Geometry check sheet. Reference: drawing and pictorial views, mm from the part's lowest x, y, z. A direction names the side the tool comes from. Round coordinates to 2 decimals unless told otherwise and drop trailing zeros. Order: outer loops, then holes, each group sorted by start corner. A loop starts at its lowest first (then second) coordinate and runs counter-clockwise, first axis right, second up.
(1) Sectioned sample at B-B, the plane y = 10. Enter the section's corners in (x, z).
(2) Tool access check on the marked faces 5 and 6. Record the directions out of +Z, -Z, +X, -X, +Y, -Y that give a thin tool (end or side, any length) a straight path to the whole face; none if there is none.
(3) Mould release check, pull along Z, two halves, no side actions. Record for the marked faces 1, 2, 3 and 4: released by +Z, released by -Z, zero draft, split by the parting line, or undercut.
(4) Depth check by flat-ended pin: pin 1 (2 mm diameter, centred on x = 4.5, z = 6, fed in from +Y); pin 2 (1.5 mm diameter, centred on y = 6.5, z = 1.5, fed in from +X). Enter the tip coordinate at first touch or a pass-through.
(5) Sectioned sample at D-D, the plane z = 1. Enter the section's corners in (x, y).
(6) Thickness scan on probe 1 along X at (y, z) = (0.65, 5); probe 2 along Z at (x, y) = (1.2, 10); probe 3 along X at (y, z) = (12.75, 9). Record the ranges inside material, lowest first.
(7) Sectioned sample at A-A, the plane z = 5. Enter the section's corners in (x, y), and give its area (3 significant figures).
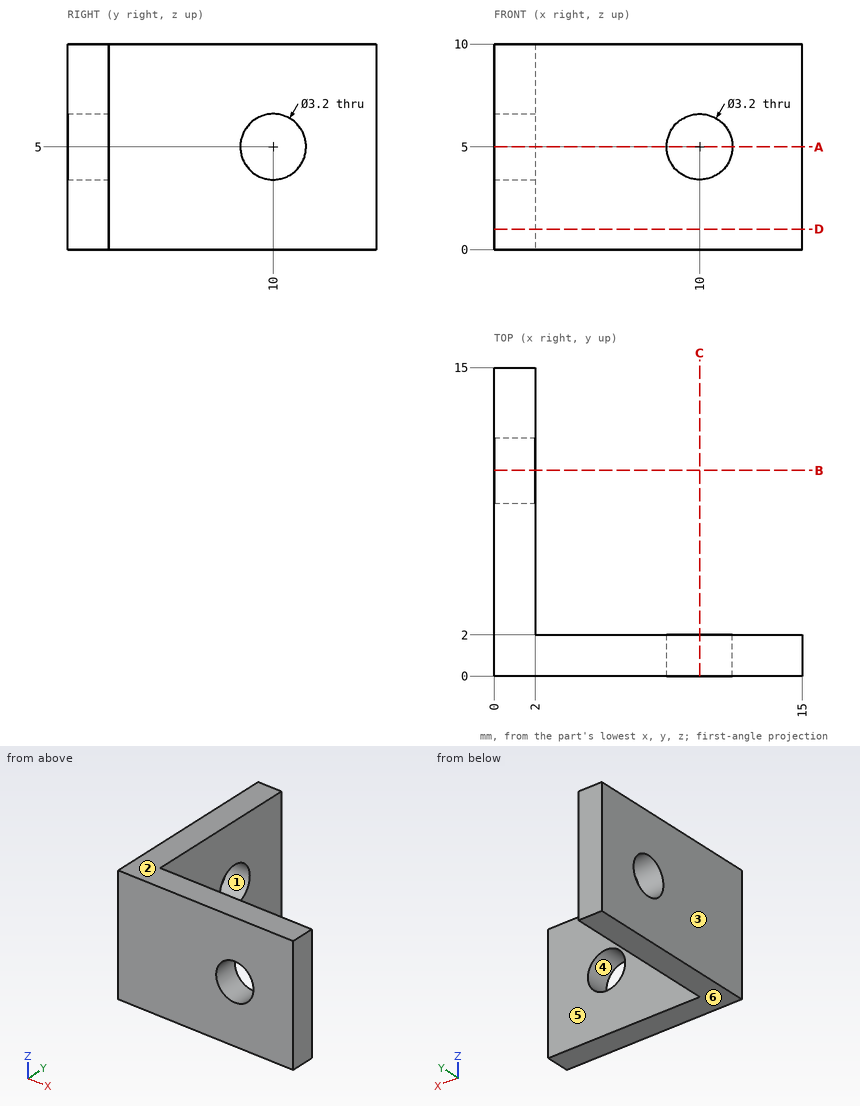
Derived:
1. outline: (0, 0) - (2, 0) - (2, 3.4) - (0, 3.4) - close; (0, 6.6) - (2, 6.6) - (2, 10) - (0, 10) - close
2. face 5: +Z, -Z, +X, +Y
2. face 6: -Z, +X, -X, +Y, -Y
3. face 1: undercut
3. face 2: released by +Z
3. face 3: zero draft
3. face 4: undercut
4. pin 1: stops at y = 2
4. pin 2: stops at x = 2
5. outline: (0, 0) - (15, 0) - (15, 2) - (2, 2) - (2, 15) - (0, 15) - close
6. probe 1: x = 0 to 8.4, 11.6 to 15
6. probe 2: z = 0 to 3.4, 6.6 to 10
6. probe 3: x = 0 to 2
7. outline: (0, 0) - (8.4, 0) - (8.4, 2) - (2, 2) - (2, 8.4) - (0, 8.4) - close; (0, 11.6) - (2, 11.6) - (2, 15) - (0, 15) - close; (11.6, 0) - (15, 0) - (15, 2) - (11.6, 2) - close
7. area: 43.2 mm2
